Design review of the part shown in the three views and the two pictorial views. Dimensions are in mm from the part's minimum x, y and z. A direction names the side the tool comes from. Round coordinates to 2 decimals unless told otherwise and drop trailing zeros. Loops run counter-clockwise (first coordinate to the right, second up) from the corner with the lowest first, then second, coordinate; pieces in that order, holes last. Notation, with made-up numbers: M -11,23.5 L 7,23.5 A27 cw 7,41.5 Z; hole C -12.5,19.25 d11. An arc over 180 degrees is marked long. Return JSON: item names as keys, results as strings. Group by question number.
Q1. For the marked faces 1 and 2, list the 3-axis set-ups (+Z, -Z, +X, -X, +Y, -Y) from which the entire face can be reached by the end or side of a thin tool; tool diameter is ignored.
Q2. Draft analysis for pull direction X (two halves, no side actions). For the marked faces 3, 4 and 5, state which applies: pulls with the +X half, pulls with the -X half, needs draft (parallel to the pull), parting line crosses it, or undercut.
Q3. Consider section C-C (x = 47.5). State the section outline as (y, z) points.
Q4. Consider section A-A (y = 26). State the section outline as (x, z) points.
Q5. Clearance check with flat-ended pins moving along their axes: pin 1 Ø1.8 at (y, z) = (10, 6.5) entering from -X; pin 2 Ø4 at (y, z) = (50.5, 4) entering from +X; pin 3 Ø3 at (x, y) = (39.5, 38.5) entering from -Z; pin 4 Ø3.5 at (y, z) = (33, 3) entering from +X. State where each tip first meets the part, or that it passes through.
Q6. Consider section D-D (y = 3). State the section outline as (x, z) points.
Q7. To check wall thickness, follow line 1 along X through (y, z) = (57.5, 4.25); line 2 along Y through (x, z) = (44.5, 8) (1 decimal); line 3 along Y through (x, z) = (31.5, 7). State the ranges of each line that lie inside material, in increasing order.
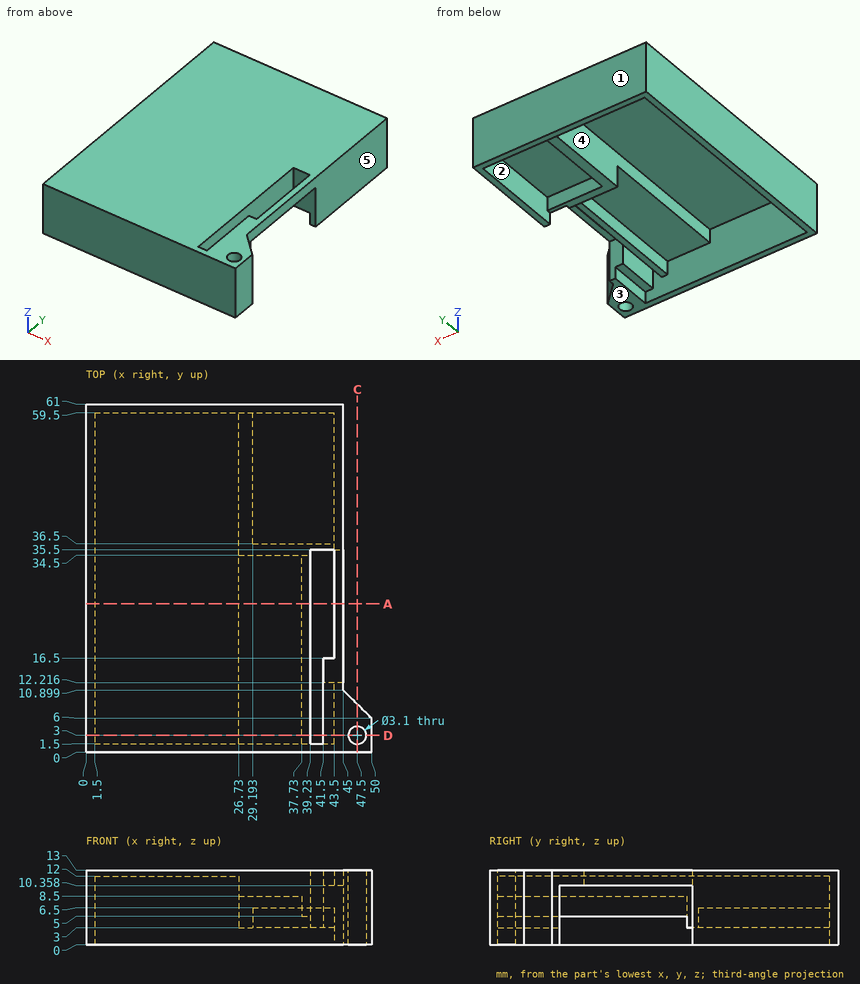
Values:
{
 "1": {"face 1": "+Z, -Z, +X, -X, +Y", "face 2": "-Z"},
 "2": {"face 3": "needs draft", "face 4": "undercut", "face 5": "pulls with the +X half"},
 "3": {"outline": "M 0,0 L 1.45,0 L 1.45,13 L 0,13 Z; M 4.55,0 L 8.45,0 L 8.45,13 L 4.55,13 Z"},
 "4": {"outline": "M 0,0 L 1.5,0 L 1.5,12 L 26.73,12 L 26.73,8.5 L 37.73,8.5 L 37.73,5 L 39.23,5 L 39.23,13 L 0,13 Z; M 43.5,10.36 L 45,10.36 L 45,13 L 43.5,13 Z"},
 "5": {"pin 1": "stops at x = 0", "pin 2": "stops at x = 45", "pin 3": "stops at z = 6.5", "pin 4": "stops at x = 39.23"},
 "6": {"outline": "M 0,0 L 1.5,0 L 1.5,12 L 26.73,12 L 26.73,8.5 L 37.73,8.5 L 37.73,5 L 39.23,5 L 39.23,13 L 0,13 Z; M 41.5,3 L 43.5,3 L 43.5,0 L 45.95,0 L 45.95,13 L 41.5,13 Z; M 49.05,0 L 50,0 L 50,13 L 49.05,13 Z"},
 "7": {"line 1": "x = 0 to 1.5, 26.73 to 29.19, 43.5 to 45", "line 2": "y = 0 to 12.2, 35.5 to 61", "line 3": "y = 0 to 1.5, 34.5 to 61"}
}
